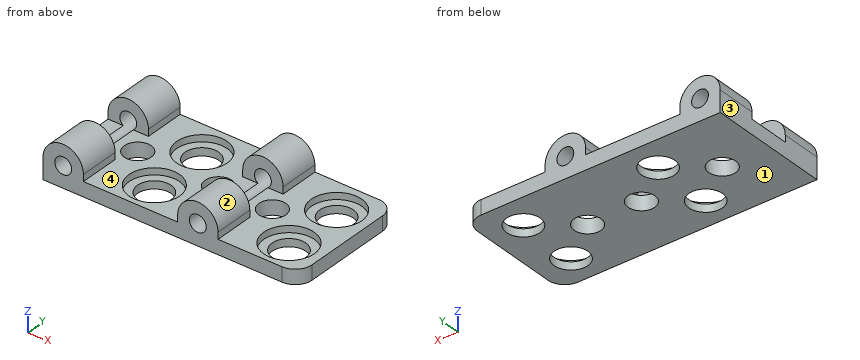
```python
from build123d import *

# Parameters (mm, degrees)
SKETCH1_R             = 6
SKETCH1_R_2           = 2.501
BOSS_EXTRUDE1_DEPTH   = 36.6
BOSS_EXTRUDE1_2_DEPTH = 36.6
BOSS_EXTRUDE2_DEPTH   = 36.6
SKETCH2_R             = 5
CUT_EXTRUDE1_DEPTH    = 60.120639374
SKETCH6_W             = 28
SKETCH6_H             = 36.6
SKETCH6_R             = 7.5
SKETCH6_W_2           = 24
BOSS_EXTRUDE3_DEPTH   = 2
FILLET2_R             = 5
SKETCH7_R             = 4
CUT_EXTRUDE2_DEPTH    = 60.325879682
SKETCH8_W             = 12
SKETCH8_H             = 12.6
CUT_EXTRUDE3_DEPTH    = 60.325879682


with BuildPart() as part:
    # Sketch1 → Boss-Extrude1 (new body)
    with BuildSketch(Plane(origin=(0, 0, 0), x_dir=(1, 0, 0), z_dir=(0, 1, 0))):
        with Locations(Location((-40, 0, 0), (0, 0, 270))):
            Circle(SKETCH1_R)
        with Locations(Location((-40, 0, 0), (0, 0, 270))):
            Circle(SKETCH1_R_2, mode=Mode.SUBTRACT)
    extrude(amount=BOSS_EXTRUDE1_DEPTH)



with BuildPart() as body_2:
    # Sketch1 → Boss-Extrude1 2 (new body)
    with BuildSketch(Plane(origin=(0, 0, 0), x_dir=(1, 0, 0), z_dir=(0, 1, 0))):
        with Locations(Location((0, 0, 0), (0, 0, 270))):
            Circle(SKETCH1_R)
        with Locations(Location((0, 0, 0), (0, 0, 270))):
            Circle(SKETCH1_R_2, mode=Mode.SUBTRACT)
    extrude(amount=BOSS_EXTRUDE1_2_DEPTH)


with BuildPart() as part_1:
    add(part.part)

    add(body_2.part)  # Boss-Extrude2 merges body 2
    # Sketch3 → Boss-Extrude2 (add)
    with BuildSketch(Plane(origin=(0, 0, 0), x_dir=(1, 0, 0), z_dir=(0, 1, 0))):
        with BuildLine():
            Line((-34, 0), (-34, 4))
            Line((-34, 4), (-6, 4))
            Line((-6, 4), (-6, 0))
            ThreePointArc((-6, 0), (0, 6), (6, 0))
            Line((6, 0), (6, 4))
            Line((6, 4), (30, 4))
            Line((30, 4), (30, 6.3))
            Line((30, 6.3), (6, 6.3))
            Line((6, 6.3), (-46, 6.3))
            Line((-46, 6.3), (-46, 0))
            ThreePointArc((-46, 0), (-40, 6), (-34, 0))
        make_face()
    extrude(amount=BOSS_EXTRUDE2_DEPTH)

    # Sketch2 → Cut-Extrude1 (cut, through all)
    with BuildSketch(Plane.XY):
        with Locations((-20, 27)):
            Circle(SKETCH2_R)
        with Locations((-20, 9)):
            Circle(SKETCH2_R)
        with Locations((20, 27)):
            Circle(SKETCH2_R)
        with Locations((20, 9)):
            Circle(SKETCH2_R)
    extrude(amount=-CUT_EXTRUDE1_DEPTH, mode=Mode.SUBTRACT)

    # Sketch6 → Boss-Extrude3 (add)
    # profile 1 of 2: a face of its own
    with BuildSketch(Plane.XY.offset(-4)):
        with Locations((-20, 18.3)):
            Rectangle(SKETCH6_W, SKETCH6_H)
        with Locations((-20, 27)):
            Circle(SKETCH6_R, mode=Mode.SUBTRACT)
        with Locations((-20, 9)):
            Circle(SKETCH6_R, mode=Mode.SUBTRACT)
    # profile 2 of 2: a face of its own
    with BuildSketch(Plane.XY.offset(-4)):
        with Locations((18, 18.3)):
            Rectangle(SKETCH6_W_2, SKETCH6_H)
        with Locations((20, 27)):
            Circle(SKETCH6_R, mode=Mode.SUBTRACT)
        with Locations((20, 9)):
            Circle(SKETCH6_R, mode=Mode.SUBTRACT)
    extrude(amount=BOSS_EXTRUDE3_DEPTH)

    # Fillet2
    fillet2_edges = [part_1.edges().sort_by_distance(p)[0] for p in [
        (30, 36.6, -4.15),
        (30, 0, -4.15),
    ]]
    fillet(fillet2_edges, radius=FILLET2_R)

    # Sketch7 → Cut-Extrude2 (cut, through all)
    with BuildSketch(Plane.XY.offset(-2)):
        with Locations((-32, 18)):
            Circle(SKETCH7_R)
        with Locations((-8, 18)):
            Circle(SKETCH7_R)
        with Locations((8, 18)):
            Circle(SKETCH7_R)
    extrude(amount=-CUT_EXTRUDE2_DEPTH, mode=Mode.SUBTRACT)

    # Sketch8 → Cut-Extrude3 (cut, through all)
    with BuildSketch(Plane.XY.offset(-2)):
        with Locations((0, 18.3)):
            Rectangle(SKETCH8_W, SKETCH8_H)
        with Locations((-40, 18.3)):
            Rectangle(SKETCH8_W, SKETCH8_H)
    extrude(amount=CUT_EXTRUDE3_DEPTH, mode=Mode.SUBTRACT)


solid = part_1.part
```
The listing builds one solid part. Answer for the finished solid, in the listing's coordinates (mm). Face numbers are marked on the shaded views. Give positions to 0.01 mm unless a question says otherwise; leave off trailing zeros. Order: outer loops, then holes, each group sorted by start corner. A loop starts at its lowest first (then second) coordinate and runs counter-clockwise, first axis right, second up. Notation, with made-up numbers: (87, -22.5) - (108, -22.5) arc R11 ccw to (108, -1.5) - close; hole circle Ø7 at (7.25, 35.5). An arc over 180 degrees is marked (long way). Use one line per item in the form item = value. Start each with the question number.
(1) Consider line 1 (Y direction, x = 20, z = -2.6); line 2 (Y direction, x = -20, z = -4.45); line 3 (X direction, y = 26, z = 1.25). Determine where each line is inside the solid, lowest interval first. Write a range as from..to.
(2) A cutting plane is placed at A-A, the plane x = -8. Write down the section's boundary in (y, z).
(3) A cutting plane is placed at C-C, the plane z = -4.75. Write down the section's boundary in (x, y).
(4) A cutting plane is placed at D-D, the plane y = 27. Write down the section's boundary in (x, z).
(5) A cutting plane is placed at B-B, the plane y = 18. Write down the section's boundary in (x, z).
(6) The mould has two halves that part along X. Classify the marked faces 1, 2, 3 and 4: released by +X, released by -X, zero draft, split by the parting line, or undercut.
(7) Flat-ended cylindrical pins translate along their axes: pin 1 Ø14 at (x, y) = (19.5, 12) entering from +Z; pin 2 Ø1 at (y, z) = (28.5, -1) entering from +X; pin 3 Ø13 at (x, y) = (8, 18) entering from -Z. Find the tip coordinate at first contact, or state that the pin passes through.
Ans:
q1.line_1 = 0..1.5, 16.5..19.5, 34.5..36.6
q1.line_2 = 0..4, 14..22, 32..36.6
q1.line_3 = -45.87..-42.17, -37.83..-34.13, -5.87..-2.17, 2.17..5.87
q2.outline = (0, -6.3) - (14, -6.3) - (14, -2) - (0, -2) - close; (22, -6.3) - (36.6, -6.3) - (36.6, -2) - (22, -2) - close
q3.outline = (-46, 0) - (25, 0) arc R5 ccw to (30, 5) - (30, 31.6) arc R5 ccw to (25, 36.6) - (-46, 36.6) - close; hole circle Ø8 at (-32, 18); hole circle Ø10 at (-20, 9); hole circle Ø10 at (-20, 27); hole circle Ø8 at (-8, 18); hole circle Ø8 at (8, 18); hole circle Ø10 at (20, 9); hole circle Ø10 at (20, 27)
q4.outline = (-46, -6.3) - (-25, -6.3) - (-25, -4) - (-27.5, -4) - (-27.5, -2) - (-34, -2) - (-34, 0) arc R6 ccw to (-46, 0) - close; (-15, -6.3) - (15, -6.3) - (15, -4) - (12.5, -4) - (12.5, -2) - (6, -2) - (6, 0) arc R6 ccw to (-6, 0) - (-6, -2) - (-12.5, -2) - (-12.5, -4) - (-15, -4) - close; (25, -6.3) - (30, -6.3) - (30, -2) - (27.5, -2) - (27.5, -4) - (25, -4) - close; hole circle Ø5 at (-40, 0); hole circle Ø5 at (0, 0)
q5.outline = (-46, -6.3) - (-36, -6.3) - (-36, -2) - (-38.5, -2) arc R2.5 cw to (-41.5, -2) - (-46, -2) - close; (-28, -6.3) - (-12, -6.3) - (-12, -2) - (-28, -2) - close; (-4, -6.3) - (4, -6.3) - (4, -2) - (1.5, -2) arc R2.5 cw to (-1.5, -2) - (-4, -2) - close; (12, -6.3) - (30, -6.3) - (30, -2) - (12, -2) - close
q6.face_1 = zero draft
q6.face_2 = undercut
q6.face_3 = released by -X
q6.face_4 = undercut
q7.pin_1 = -2
q7.pin_2 = 6
q7.pin_3 = -6.3
